```python
from build123d import *

# Parameters (mm, degrees)
SKETCH_R  = 1.9
PAD_DEPTH = 2
FILLET_R  = 1


with BuildPart() as part:
    # Sketch → Pad (new body)
    with BuildSketch(Plane.XY):
        with BuildLine():
            Line((-15.000027, 10), (15.000027, 10))
            ThreePointArc((15.000027, -10), (25, 0), (15.000027, 10))
            Line((15.000027, -10), (-15.000027, -10))
            ThreePointArc((-15.000027, 10), (-25, 0), (-15.000027, -10))
        make_face()
        with Locations((-15, 0)):
            Circle(SKETCH_R, mode=Mode.SUBTRACT)
        with Locations((15, 0)):
            Circle(SKETCH_R, mode=Mode.SUBTRACT)
        with BuildLine():
            ThreePointArc((-0.966331, 5.718934), (0, 5.35), (0.966331, 5.718934))
            Line((0.966331, 5.718934), (2.579727, 5.19471))
            ThreePointArc((2.579727, 5.19471), (3.144651, 4.328241), (4.143283, 4.058719))
            Line((4.143283, 4.058719), (5.140417, 2.686283))
            ThreePointArc((5.140417, 2.686283), (5.088152, 1.653241), (5.737642, 0.848212))
            Line((5.737642, 0.848212), (5.737642, -0.848212))
            ThreePointArc((5.737642, -0.848212), (5.088152, -1.653241), (5.140417, -2.686283))
            Line((4.143283, -4.058719), (5.140417, -2.686283))
            ThreePointArc((4.143283, -4.058719), (3.144651, -4.328241), (2.579727, -5.19471))
            Line((0.966331, -5.718934), (2.579727, -5.19471))
            ThreePointArc((0.966331, -5.718934), (0, -5.35), (-0.966331, -5.718934))
            Line((-2.579727, -5.19471), (-0.966331, -5.718934))
            ThreePointArc((-2.579727, -5.19471), (-3.144651, -4.328241), (-4.143283, -4.058719))
            Line((-5.140417, -2.686283), (-4.143283, -4.058719))
            ThreePointArc((-5.140417, -2.686283), (-5.088152, -1.653241), (-5.737642, -0.848212))
            Line((-5.737642, 0.848212), (-5.737642, -0.848212))
            ThreePointArc((-5.737642, 0.848212), (-5.088152, 1.653241), (-5.140417, 2.686283))
            Line((-5.140417, 2.686283), (-4.143283, 4.058719))
            ThreePointArc((-4.143283, 4.058719), (-3.144651, 4.328241), (-2.579727, 5.19471))
            Line((-2.579727, 5.19471), (-0.966331, 5.718934))
        make_face(mode=Mode.SUBTRACT)
    extrude(amount=PAD_DEPTH)

    # Fillet
    fillet_edges = [part.edges().sort_by_distance(p)[0] for p in [
        (0, -10, 2),
        (-25, 0, 2),
        (0, 10, 2),
        (25, 0, 2),
    ]]
    fillet(fillet_edges, radius=FILLET_R)


solid = part.part
```
Verification items for the finished model (mm, model axes). A direction names the side the tool comes from. Give positions to 0.01 mm unless a question says otherwise; leave off trailing zeros. Order: outer loops, then holes, each group sorted by start corner. A loop starts at its lowest first (then second) coordinate and runs counter-clockwise, first axis right, second up. Notation, with made-up numbers: (30.25, 61) -> (54.25, 61) arc R5 cw to (54.25, 67) -> close; hole circle Ø1 at (22.25, 21.25). An arc over 180 degrees is marked (long way). One line per item, written item: value.
(1) Sectioned sample at B-B on x = 0. Record the cut outline in (y, z).
Final values:
outline: (-10, 0) -> (-5.35, 0) -> (-5.35, 2) -> (-9, 2) arc R1 ccw to (-10, 1) -> close; (5.35, 0) -> (10, 0) -> (10, 1) arc R1 ccw to (9, 2) -> (5.35, 2) -> close
(2) Sectioned sample at A-A on y = 0. Record the cut outline in (x, z), then the cut area to 3 significant figures.
Final values:
outline: (-25, 0) -> (-16.9, 0) -> (-16.9, 2) -> (-24, 2) arc R1 ccw to (-25, 1) -> close; (-13.1, 0) -> (-5.74, 0) -> (-5.74, 2) -> (-13.1, 2) -> close; (5.74, 0) -> (13.1, 0) -> (13.1, 2) -> (5.74, 2) -> close; (16.9, 0) -> (25, 0) -> (25, 1) arc R1 ccw to (24, 2) -> (16.9, 2) -> close
area: 61.4 mm^2
(3) Draft check along X on faces 3 (the face through (0.2, -10, 0.5)), 4 (the face through (-25, 0.2, 0.5)), 5 (the face through (-1.784, -5.453, 0.986)). Enter one of: pulls with the +X half, pulls with the -X half, needs draft (parallel to the pull), parting line crosses it, or undercut.
Final values:
face 3: needs draft
face 4: pulls with the -X half
face 5: undercut
(4) Tool access check on faces 1 (the face through (-3.157, 4.32, 0.986)), 2 (the face through (-0.2, 10, 0.5)). Record the directions out of +Z, -Z, +X, -X, +Y, -Y that give a thin tool (end or side, any length) a straight path to the whole face; none if there is none.
Final values:
face 1: +Z, -Z
face 2: +Z, -Z, +X, -X, +Y
(5) Scan lines: line 1 along Y through (x, z) = (15, 0.55); line 2 along X through (y, z) = (1, 1.1); line 3 along Y through (x, z) = (11, 1.1). Record each from-to range of solid material in increasing order. Write a range as [from, to].
Final values:
line 1: [-10, -1.9], [1.9, 10]
line 2: [-24.94, -16.62], [-13.38, -5.52], [5.52, 13.38], [16.62, 24.94]
line 3: [-9.99, 9.99]
(6) Gauge pin test, flat end, axial feed: pin 1 (6 mm diameter, centred on x = 15, y = 0, fed in from +Z). Record the tip position at first contact, or that the pin passes through.
Final values:
pin 1: z = 2
